Can you work these out from the model? Positions are in its coordinate system, mm. A direction names the side the tool comes from. Coordinates: 2 decimals unless noted, no trailing zeros. Order: outer loops, then holes, each group sorted by start corner. A loop starts at its lowest first (then second) coordinate and runs counter-clockwise, first axis right, second up. Notation, with made-up numbers: (-5, 17) -> (36, 17) arc R12 ccw to (36, 21) -> close; hole circle Ø4 at (-35.75, 59). An arc over 180 degrees is marked (long way). Write item = value, one per line.
```python
from build123d import *

# Parameters (mm, degrees)
EXTRUDE_1_DEPTH     = 3
SKETCH_2_W          = 80
SKETCH_2_H          = 2.7
CUT_EXTRUDE_1_DEPTH = 3
SKETCH_3_W          = 100
SKETCH_3_H          = 8
EXTRUDE_3_DEPTH     = 3
SKETCH_4_W          = 3
SKETCH_4_H          = 5.5
CUT_EXTRUDE_2_DEPTH = 3


with BuildPart() as part:
    # 草圖1 → 填料-伸長1 (new body)
    with BuildSketch(Plane.XY):
        Polygon((-61.919288793, 23.718072979), (-52.919288793, 23.718072979), (-52.919288793, 26.718072979), (-42.919288793, 26.718072979), (-42.919288793, 23.718072979), (-28.919288793, 23.718072979), (-28.919288793, 26.718072979), (-18.919288793, 26.718072979), (-18.919288793, 23.718072979), (-4.919288793, 23.718072979), (-4.919288793, 26.718072979), (5.080711207, 26.718072979), (5.080711207, 23.718072979), (19.080711207, 23.718072979), (19.080711207, 26.718072979), (29.080711207, 26.718072979), (29.080711207, 23.718072979), (38.080711207, 23.718072979), (38.080711207, 16.218072979), (35.080711207, 16.218072979), (35.080711207, 6.218072979), (38.080711207, 6.218072979), (38.080711207, -3.781927021), (35.080711207, -3.781927021), (35.080711207, -13.781927021), (38.080711207, -13.781927021), (38.080711207, -23.781927021), (35.080711207, -23.781927021), (35.080711207, -33.781927021), (38.080711207, -33.781927021), (38.080711207, -41.281927021), (29.080711207, -41.281927021), (29.080711207, -44.281927021), (19.080711207, -44.281927021), (19.080711207, -41.281927021), (5.080711207, -41.281927021), (5.080711207, -44.281927021), (-4.919288793, -44.281927021), (-4.919288793, -41.281927021), (-18.919288793, -41.281927021), (-18.919288793, -44.281927021), (-28.919288793, -44.281927021), (-28.919288793, -41.281927021), (-42.919288793, -41.281927021), (-42.919288793, -44.281927021), (-52.919288793, -44.281927021), (-52.919288793, -41.281927021), (-61.919288793, -41.281927021), (-61.919288793, -33.781927021), (-58.919288793, -33.781927021), (-58.919288793, -23.781927021), (-61.919288793, -23.781927021), (-61.919288793, -13.781927021), (-58.919288793, -13.781927021), (-58.919288793, -3.781927021), (-61.919288793, -3.781927021), (-61.919288793, 6.218072979), (-58.919288793, 6.218072979), (-58.919288793, 16.218072979), (-61.919288793, 16.218072979), align=None)
    extrude(amount=EXTRUDE_1_DEPTH)

    # 草圖2 → 除料-伸長1 (cut)
    with BuildSketch(Plane(origin=(0, 0, 0), x_dir=(-1, 0, 0), z_dir=(0, 0, -1))):
        with Locations((11.919288793, -8.781927021)):
            Rectangle(SKETCH_2_W, SKETCH_2_H)
        with Locations((11.919288793, 6.218072979)):
            Rectangle(SKETCH_2_W, SKETCH_2_H)
        with Locations((11.919288793, -23.781927021)):
            Rectangle(SKETCH_2_W, SKETCH_2_H)
    extrude(amount=-CUT_EXTRUDE_1_DEPTH, mode=Mode.SUBTRACT)

    # 草圖3 → 填料-伸長3 (add)
    with BuildSketch(Plane.XY.offset(3)):
        with Locations((-11.919288793, 27.718072979)):
            Rectangle(SKETCH_3_W, SKETCH_3_H)
    extrude(amount=-EXTRUDE_3_DEPTH)

    # 草圖4 → 除料-伸長2 (cut)
    with BuildSketch(Plane.XY.offset(3)):
        with Locations((36.580711207, 28.968072979)):
            Rectangle(SKETCH_4_W, SKETCH_4_H)
        with Locations((-60.419288793, 28.968072979)):
            Rectangle(SKETCH_4_W, SKETCH_4_H)
    extrude(amount=-CUT_EXTRUDE_2_DEPTH, mode=Mode.SUBTRACT)


solid = part.part
```
Item 1: If I drill on probe 1 along Y at (x, z) = (13.5, 1.55); probe 2 along Y at (x, z) = (-24.5, 1.35); probe 3 along X at (y, z) = (-29, 1.9), over which ranges is the centre line in solid material (lowest first)?
A:
probe_1 = -41.28 to -25.13, -22.43 to -10.13, -7.43 to 4.87, 7.57 to 31.72
probe_2 = -44.28 to -25.13, -22.43 to -10.13, -7.43 to 4.87, 7.57 to 31.72
probe_3 = -58.92 to 35.08
Item 2: For faces 5 (the flat face through (-28.919, -43, 1)), 6 (the flat face through (37, -23.782, 1)), 7 (the flat face through (37, 26.218, 2)), 8 (the flat face through (28.081, -24, 1)), which set-ups out of +Z, -Z, +X, -X, +Y, -Y let a thin tool reach every point of the face, with its end or its side?
A:
face_5 = +Z, -Z, -Y
face_6 = +Z, -Z, +X
face_7 = +Z, -Z, +X, +Y
face_8 = +Z, -Z
Item 3: I'm going to push flat-ended pins straight in: P1, Ø0.9, axis at x = 36.5, z = 2, coming from the +Y side; P2, Ø0.9, axis at y = -28, z = 1, coming from the -X side; P3, Ø0.9, axis at x = 36, z = 1, coming from the -Y side. Where does each tip first touch, or does it pass through?
A:
P1 = 26.22
P2 = -58.92
P3 = -41.28
Item 4: I want a section at B-B, the plane z = 2.55. Give the number of separate pieces and of enclosed holes in the cut face, plus the area to 3 significant figures.
A:
separate_pieces = 1
enclosed_holes = 3
area = 6,560 mm2
Item 5: If we mould it in two halves opening along X, with no side actions, what happens to faces 1 (the flat face through (29.081, -43, 1)), 2 (the flat face through (37, -3.782, 1)), 3 (the flat face through (-51.919, 6, 1)), 4 (the flat face through (-52.919, -43, 1))? For each: pulls with the +X half, pulls with the -X half, needs draft (parallel to the pull), parting line crosses it, or undercut.
A:
face_1 = pulls with the +X half
face_2 = needs draft
face_3 = undercut
face_4 = pulls with the -X half
Item 6: I want a section at A-A, the plane x = -48. Please give me the cut outline in (y, z).
A:
outline = (-44.28, 0) -> (-25.13, 0) -> (-25.13, 3) -> (-44.28, 3) -> close; (-22.43, 0) -> (-10.13, 0) -> (-10.13, 3) -> (-22.43, 3) -> close; (-7.43, 0) -> (4.87, 0) -> (4.87, 3) -> (-7.43, 3) -> close; (7.57, 0) -> (31.72, 0) -> (31.72, 3) -> (7.57, 3) -> close
Item 7: I want a section at D-D, the plane y = -29. Please give me the cut outline in (x, z), plus the area to 3 significant figures.
A:
outline = (-58.92, 0) -> (35.08, 0) -> (35.08, 3) -> (-58.92, 3) -> close
area = 282 mm2
Item 8: I want a section at C-C, the plane x = 7. Please give me the cut outline in (y, z).
A:
outline = (-41.28, 0) -> (-25.13, 0) -> (-25.13, 3) -> (-41.28, 3) -> close; (-22.43, 0) -> (-10.13, 0) -> (-10.13, 3) -> (-22.43, 3) -> close; (-7.43, 0) -> (4.87, 0) -> (4.87, 3) -> (-7.43, 3) -> close; (7.57, 0) -> (31.72, 0) -> (31.72, 3) -> (7.57, 3) -> close
